from build123d import *

# Parameters (mm, degrees)
ESQUISSE1_R                  = 36.75
EXTRUSION1_DEPTH             = 1
ENL_V_MAT_EXTRU_1_DEPTH      = 2
R_P_TITION_CIRCULAIRE1_COUNT = 18
ESQUISSE3_R                  = 21
EXTRUSION2_DEPTH             = 2.125
ESQUISSE4_R                  = 16
ENL_V_MAT_EXTRU_2_DEPTH      = 3.125
ENL_V_MAT_EXTRU_2_DEPTH_BACK = 3.125
CHANFREIN1_SIZE              = 0.5


with BuildPart() as part:
    # Esquisse1 → Extrusion1 (new body, symmetric)
    with BuildSketch(Plane.XY):
        Circle(ESQUISSE1_R)
    extrude(amount=EXTRUSION1_DEPTH, both=True)

    # Esquisse2 → Enlèv. mat.-Extru.1 (cut, symmetric)
    with BuildSketch(Plane.XY):
        with BuildLine():
            Line((-5.312971291, 36.363922177), (-3.276608177, 33.455694255))
            ThreePointArc((-3.276608177, 33.455694255), (0.987178532, 31.873728783), (3.974883244, 35.302447552))
            Line((3.974883244, 35.302447552), (4.111888112, 36.519239808))
            ThreePointArc((4.111888112, 36.519239808), (-0.605541982, 36.745010803), (-5.312971291, 36.363922177))
        make_face()
    enl_v_mat_extru_1 = extrude(amount=ENL_V_MAT_EXTRU_1_DEPTH, both=True, mode=Mode.SUBTRACT)

    # Répétition circulaire1: Enlèv. mat.-Extru.1 ×18 about axis
    r_p_tition_circulaire1_axis = Axis((0, 0, 0), (0, 0, 1))
    for i in range(1, R_P_TITION_CIRCULAIRE1_COUNT):
        add(enl_v_mat_extru_1.rotate(r_p_tition_circulaire1_axis, i * 360 / R_P_TITION_CIRCULAIRE1_COUNT), mode=Mode.SUBTRACT)

    # Esquisse3 → Extrusion2 (add, symmetric)
    with BuildSketch(Plane.XY):
        Circle(ESQUISSE3_R)
    extrude(amount=EXTRUSION2_DEPTH, both=True)

    # Esquisse4 → Enlèv. mat.-Extru.2 (cut, two sides)
    with BuildSketch(Plane.XY) as enl_v_mat_extru_2_sk:
        Circle(ESQUISSE4_R)
    extrude(amount=ENL_V_MAT_EXTRU_2_DEPTH, mode=Mode.SUBTRACT)
    extrude(enl_v_mat_extru_2_sk.sketch, amount=-ENL_V_MAT_EXTRU_2_DEPTH_BACK, mode=Mode.SUBTRACT)

    # Chanfrein1
    chanfrein1_edges = [part.edges().sort_by_distance(p)[0] for p in [
        (-21, 0, -2.125),
        (-21, 0, 2.125),
        (-16, 0, -2.125),
        (-16, 0, 2.125),
    ]]
    chamfer(chanfrein1_edges, length=CHANFREIN1_SIZE)


solid = part.part
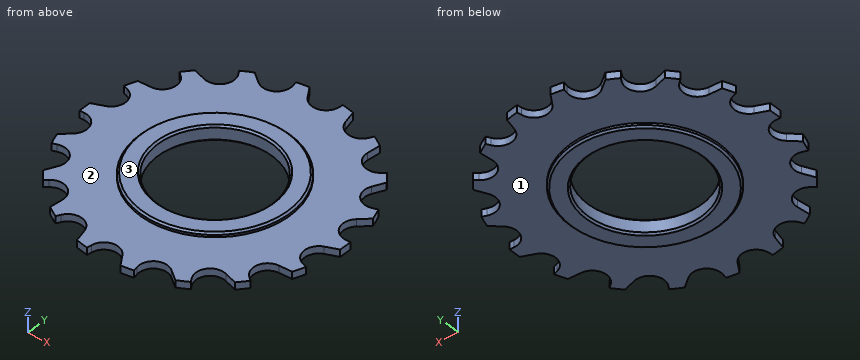
Input: part model. Units: mm. Frame: model coordinates. Face numbers are marked on the shaded views. A direction names the side the tool comes from. Coordinates: 2 decimals unless noted, no trailing zeros. Order: outer loops, then holes, each group sorted by start corner. A loop starts at its lowest first (then second) coordinate and runs counter-clockwise, first axis right, second up. Notation, with made-up numbers: M 81.5,81 L 131.5,81 A18 ccw 131.5,106 Z; hole C 80.25,51 d2. An arc over 180 degrees is marked long. One line per question, with ' | ' between items.
Item 1: Pin query (flat end, axial travel): pin 1 (1 mm diameter, centred on y = -17, z = 1, fed in from -X); pin 2 (12 mm diameter, centred on x = 28, y = -7.5, fed in from +Z); pin 3 (1 mm diameter, centred on x = 3, z = 0, fed in from +Y). Return the tip coordinate at first contact, or that it passes through.
Geometry results:
pin 1: stops at x = -27.2 | pin 2: stops at z = 1 | pin 3: stops at y = 33.81
Item 2: Section A-A (x = 0). Output: boundary loops of the cut face in (y, z) (3 decimals).
Geometry results:
outline: M -31.75,-1 L -21,-1 L -21,-1.625 L -20.5,-2.125 L -16.5,-2.125 L -16,-1.625 L -16,1.625 L -16.5,2.125 L -20.5,2.125 L -21,1.625 L -21,1 L -31.75,1 Z; M 16,-1.625 L 16.5,-2.125 L 20.5,-2.125 L 21,-1.625 L 21,-1 L 31.75,-1 L 31.75,1 L 21,1 L 21,1.625 L 20.5,2.125 L 16.5,2.125 L 16,1.625 Z
Item 3: Reachability of the marked faces 1, 2 and 3 from +Z, -Z, +X, -X, +Y, -Y: full face, straight path, thin tool, end or side. Return the list, or none.
Geometry results:
face 1: -Z | face 2: +Z | face 3: +Z, +X, -X, +Y, -Y
Item 4: Ray query, line 1 along X through (y, z) = (0, 0.1); line 2 along Y through (x, z) = (0, -0.25); line 3 along X through (y, z) = (-31, -0.65). Return the intervals inside material, ascending.
Geometry results:
line 1: x = -36.75 to -16, 16 to 36.75 | line 2: y = -31.75 to -16, 16 to 31.75 | line 3: x = -19.28 to -15.27, -9.18 to 9.18, 15.5 to 19.74
Item 5: Section B-B (y = 0). Output: boundary loops of the cut face in (x, z) (3 decimals), then the cut area to 4 significant figures.
Geometry results:
outline: M -36.75,-1 L -21,-1 L -21,-1.625 L -20.5,-2.125 L -16.5,-2.125 L -16,-1.625 L -16,1.625 L -16.5,2.125 L -20.5,2.125 L -21,1.625 L -21,1 L -36.75,1 Z; M 16,-1.625 L 16.5,-2.125 L 20.5,-2.125 L 21,-1.625 L 21,-1 L 36.75,-1 L 36.75,1 L 21,1 L 21,1.625 L 20.5,2.125 L 16.5,2.125 L 16,1.625 Z | area: 104.5 mm^2
